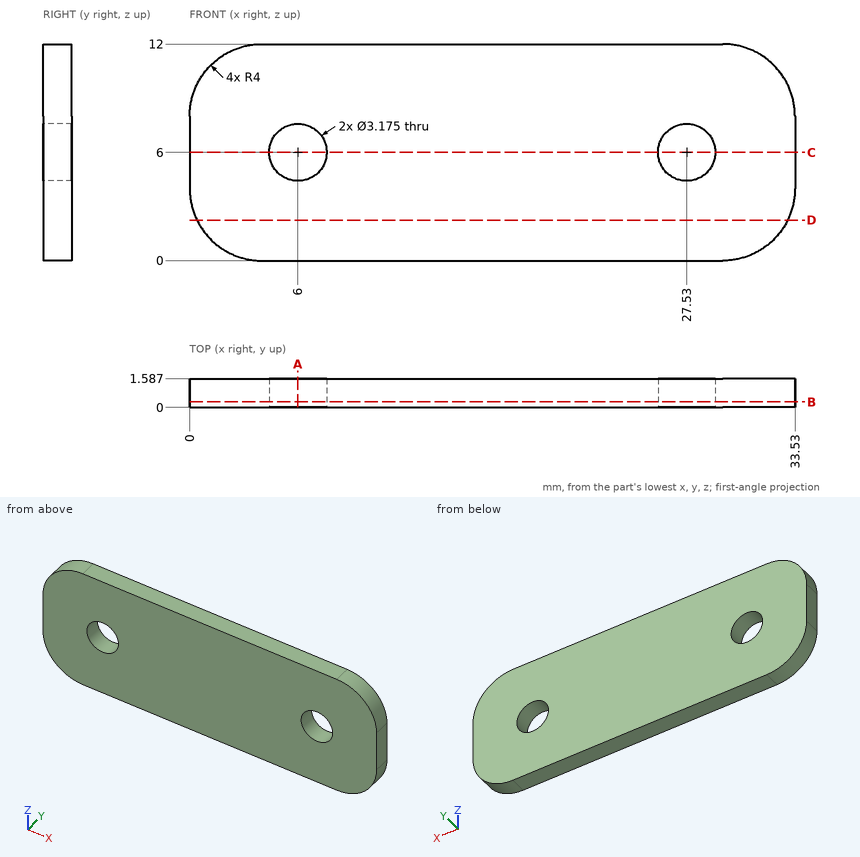
For this review, use the dimensioned drawing (mm, ordinates from the lowest corner) and the shaded views. Round coordinates to 2 decimals unless told otherwise and drop trailing zeros. Order: outer loops, then holes, each group sorted by start corner. A loop starts at its lowest first (then second) coordinate and runs counter-clockwise, first axis right, second up. Notation, with made-up numbers: M 70,-32 L 94,-32 A32 cw 94,2 Z; hole C 56.5,52 d5. An arc over 180 degrees is marked long. Write each question's results on one line, items separated by ' | '. Start each with the question number.
1. Add section C-C (z = 6). State the section outline as (x, y) points.
2. Add section B-B (y = 0.3). State the section outline as (x, z) points (1 decimal).
3. To check wall thickness, follow L1, parallel to X at y = 0.45, z = 6; L2, parallel to X at y = 0.3, z = 2.75; L3, parallel to X at y = 0.8, z = 2.25 (1 decimal). State the ranges of each line that lie inside material, in increasing order. Write a range as [from, to].
4. Add section A-A (x = 6). State the section outline as (y, z) points, then the cut area to 3 significant figures.
5. Add section D-D (z = 2.25). State the section outline as (x, y) points.
Output values:
1) outline: M 0,0 L 4.41,0 L 4.41,1.59 L 0,1.59 Z; M 7.59,0 L 25.94,0 L 25.94,1.59 L 7.59,1.59 Z; M 29.12,0 L 33.53,0 L 33.53,1.59 L 29.12,1.59 Z
2) outline: M 0,4 A4 ccw 4,0 L 29.5,0 A4 ccw 33.5,4 L 33.5,8 A4 ccw 29.5,12 L 4,12 A4 ccw 0,8 Z; hole C 6,6 d3.2; hole C 27.5,6 d3.2
3) L1: [0, 4.41], [7.59, 25.94], [29.12, 33.53] | L2: [0.2, 33.33] | L3: [0.4, 33.1]
4) outline: M 0,0 L 1.59,0 L 1.59,4.41 L 0,4.41 Z; M 0,7.59 L 1.59,7.59 L 1.59,12 L 0,12 Z | area: 14.0 mm^2
5) outline: M 0.4,0 L 33.13,0 L 33.13,1.59 L 0.4,1.59 Z
